Drawing for the job (mm, zero at the part's lowest x, y, z). A direction names the side the tool comes from. Round coordinates to 2 decimals unless told otherwise and drop trailing zeros. Write each loop counter-clockwise with the first axis right and the second up, starting at its lowest first coordinate (ties: lowest second). Pieces come first, ordered by that corner, then holes. Notation, with made-up numbers: (87, 0) - (144, 0) arc R12 ccw to (144, 23) - close; hole circle Ø4 at (81.5, 8). An arc over 180 degrees is marked (long way). One line per question, with ' | ' between items.
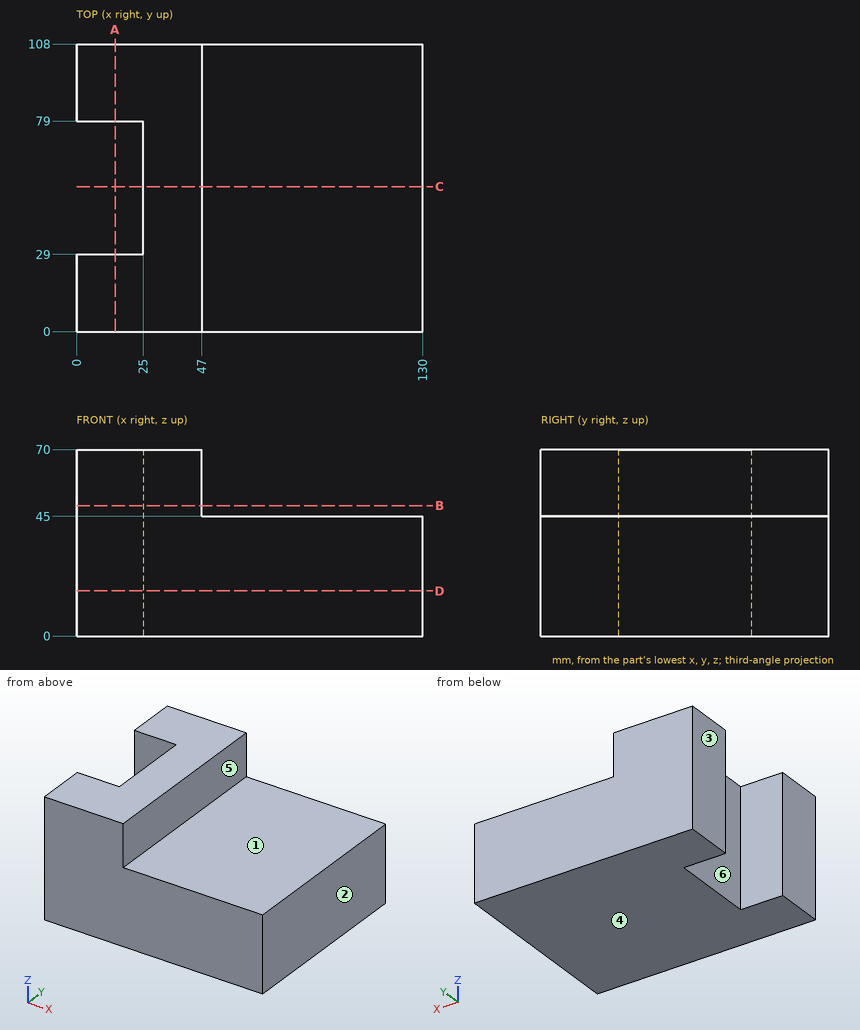
Q1. Which spindle directions (+Z, -Z, +X, -X, +Y, -Y) get a long thin tool onto all of the face, cutting with end or side? Do the marked faces 4, 5 and 6. Say none if no direction does.
Found:
face 4: -Z, +X, -X, +Y, -Y | face 5: +Z, +X, +Y, -Y | face 6: +Z, -Z, -X
Q2. Pull direction X, two halves, no side cores. Call the marked faces 1, 2 and 3: +X half, -X half, draft (parallel to the pull), parting line (faces both ways), or undercut.
Found:
face 1: draft | face 2: +X half | face 3: -X half
Q3. Saw through at C-C, the plane y = 54.5. List the corners of the cut face in (x, z).
Found:
outline: (25, 0) - (130, 0) - (130, 45) - (47, 45) - (47, 70) - (25, 70) - close
Q4. Drop flat-ended pins along their axis: pin 1 (25 mm diameter, centred on x = 96.5, y = 62, fed in from +Z); pin 2 (25 mm diameter, centred on y = 64.5, z = 51.5, fed in from -X). Give the stop position or say it passes through.
Found:
pin 1: z = 45 | pin 2: x = 25
Q5. Drill centre lines: L1, parallel to Y at x = 10, z = 66; L2, parallel to Z at x = 57, y = 48.5; L3, parallel to X at y = 23, z = 62.5. Where is each one in solid material? Low to high. Write a range as from..to.
Found:
L1: 0..29, 79..108 | L2: 0..45 | L3: 0..47
Q6. Saw through at B-B, the plane z = 49. List the corners of the cut face in (x, y), then the cut area to 3 significant figures.
Found:
outline: (0, 0) - (47, 0) - (47, 108) - (0, 108) - (0, 79) - (25, 79) - (25, 29) - (0, 29) - close | area: 3,830 mm^2
Q7. Saw through at D-D, the plane z = 17. List the corners of the cut face in (x, y), then the cut area to 3 significant figures.
Found:
outline: (0, 0) - (130, 0) - (130, 108) - (0, 108) - (0, 79) - (25, 79) - (25, 29) - (0, 29) - close | area: 12,800 mm^2
Q8. Saw through at A-A, the plane x = 14.5. List the corners of the cut face in (y, z).
Found:
outline: (0, 0) - (29, 0) - (29, 70) - (0, 70) - close; (79, 0) - (108, 0) - (108, 70) - (79, 70) - close
